from build123d import *

# Parameters (mm, degrees)
F0_W     = 63.1698
F0_H     = 25.4
F0_W_2   = 51.1302
F2_R     = 9.525
F3_DEPTH = 25.4


with BuildPart() as f1:
    # F0 (on Top) → F1 (revolve)
    with BuildSketch(Plane.XY):
        with Locations((82.7151, 12.7)):
            Rectangle(F0_W, F0_H)
        with Locations((25.5651, 12.7)):
            Rectangle(F0_W_2, F0_H)
    revolve(axis=Axis((0, 12.7, 0), (0, -1, 0)))

    # F2 (on face) → F3 (cut, through all)
    with BuildSketch(Plane.XZ):
        with Locations((-95.25, 0)):
            Circle(F2_R)
        with Locations((-67.351921, -67.351921)):
            Circle(F2_R)
        with Locations((0, -95.25)):
            Circle(F2_R)
        with Locations((67.351921, -67.351921)):
            Circle(F2_R)
        with Locations((95.25, 0)):
            Circle(F2_R)
        with Locations((67.351921, 67.351921)):
            Circle(F2_R)
        with Locations((0, 95.25)):
            Circle(F2_R)
        with Locations((-67.351921, 67.351921)):
            Circle(F2_R)
    extrude(amount=-F3_DEPTH, mode=Mode.SUBTRACT)


solid = f1.part
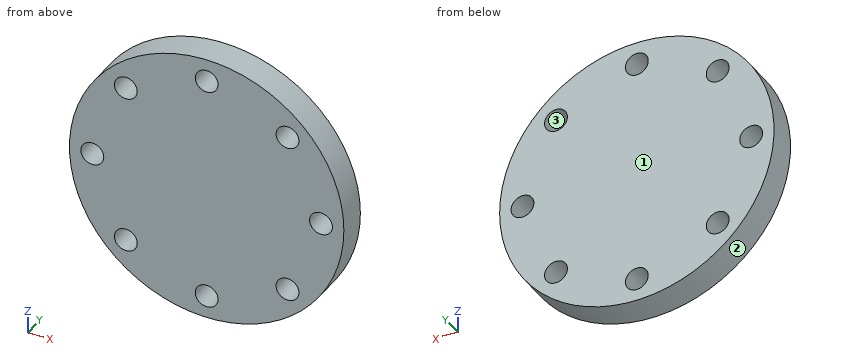
Design review of the part built by this model. Coordinates are the model's own, in mm. Face numbers are marked on the shaded views. Coordinates: 2 decimals unless noted, no trailing zeros. Order: outer loops, then holes, each group sorted by start corner. A loop starts at its lowest first (then second) coordinate and runs counter-clockwise, first axis right, second up. Notation, with made-up numbers: (8, -17) - (60, -17) arc R28 ccw to (60, 12) - close; hole circle Ø2 at (31.5, 82). An arc over 180 degrees is marked (long way). Put each result on its own line as item: value.
1) Wall thickness on L1, parallel to Z at x = 0, y = 14.5 (3 decimals); L2, parallel to Z at x = -69, y = 13; L3, parallel to X at y = 21.25, z = -96: over which ranges is each line inside the solid? List them lowest first. Write a range as from..to.
Response values:
L1: z = -114.3..-104.775, -85.725..85.725, 104.775..114.3
L2: z = -91.12..-76.73, -57.97..57.97, 76.73..91.12
L3: x = -62.04..-9.5, 9.5..62.04
2) The part is to be moulded in two halves that separate along X. For the marked faces 1, 2 and 3, say which applies: released by +X, released by -X, zero draft, split by the parting line, or undercut.
Response values:
face 1: zero draft
face 2: split by the parting line
face 3: undercut
3) Insertion check: P1, Ø3, axis at y = 13.5, z = 57, coming from the +X side; P2, Ø3, axis at x = 32, y = 21.5, coming from the +Z side; P3, Ø5, axis at x = 75, y = 3.5, coming from the +Z side. Each pin has a flat end and moves straight along its axis. Give the tip position at first contact, or say it passes through.
Response values:
P1: stops at x = 99.92
P2: stops at z = 110.16
P3: stops at z = 88.36
4) Take a section at B-B, the plane x = 0. Give the boundary of the cut face in (y, z) (3 decimals), and give its area (3 significant figures).
Response values:
outline: (0, -114.3) - (25.4, -114.3) - (25.4, -104.775) - (0, -104.775) - close; (0, -85.725) - (25.4, -85.725) - (25.4, 85.725) - (0, 85.725) - close; (0, 104.775) - (25.4, 104.775) - (25.4, 114.3) - (0, 114.3) - close
area: 4,840 mm²
5) Take a section at A-A, the plane z = 0. Give the boundary of the cut face in (x, y) (3 decimals), and give its area (3 significant figures).
Response values:
outline: (-114.3, 0) - (-104.775, 0) - (-104.775, 25.4) - (-114.3, 25.4) - close; (-85.725, 0) - (85.725, 0) - (85.725, 25.4) - (-85.725, 25.4) - close; (104.775, 0) - (114.3, 0) - (114.3, 25.4) - (104.775, 25.4) - close
area: 4,840 mm²
6) Take a section at D-D, the plane y = 5.75. Count the separate pieces of the cut face and the enclosed holes in it, and give its area (3 significant figures).
Response values:
separate pieces: 1
enclosed holes: 8
area: 38,800 mm²
7) Take a section at C-C, the plane x = -95.25. Give the boundary of the cut face in (y, z) (3 decimals), and give its area (3 significant figures).
Response values:
outline: (0, -63.182) - (25.4, -63.182) - (25.4, -9.525) - (0, -9.525) - close; (0, 9.525) - (25.4, 9.525) - (25.4, 63.182) - (0, 63.182) - close
area: 2,730 mm²
